Work out the finished part from the listing and answer in its coordinate system (mm). A direction names the side the tool comes from. Coordinates: 2 decimals unless noted, no trailing zeros. Order: outer loops, then holes, each group sorted by start corner. A loop starts at its lowest first (then second) coordinate and runs counter-clockwise, first axis right, second up. Notation, with made-up numbers: M 76.25,-14.5 L 93.25,-14.5 A29 cw 93.25,21.5 Z; hole C 29.25,46.25 d11. An arc over 180 degrees is marked long. Write item = value, one per line. Start each with the question number.
Q1. Determine the mould class of faces 5 (the flat face through (0, 28, 0)), 6 (the flat face through (0, 1000, -290)), 7 (the flat face through (0, 17, 10)) for opening direction Z: released by +Z, released by -Z, zero draft, split by the parting line, or undercut.
Q2. Straight lines are drawn through the part: line 1 along Y through (x, z) = (1.5, 45); line 2 along Z through (x, y) = (-6, 830); line 3 along Z through (x, y) = (-2, 25.5). For each, find the intervals that lie inside material, in ascending order.
Q3. Each of these flat-tipped pins is pushed along its axis until it touches: P1, Ø15, axis at x = 4.5, y = 21, coming from the +Z side; P2, Ø5, axis at x = 0.5, z = 18.5, coming from the +Y side; P3, Ø25, axis at x = 0, y = 38.5, coming from the -Z side; P4, Ø8, axis at x = -15.5, z = 32.5, coming from the -Y side. Where does it stop, or does it pass through?
Q4. Find section A-A on y = 872. Give the vertices of the cut face in (x, z), and give its area (3 significant figures).
Q5. Find section B-B on z = -135.5. Give the vertices of the cut face in (x, y).
Q6. A tool of negligible diameter and unlimited length cuts with its end or side. For faces 1 (the cylindrical face through (-2.17, 523.42, -280.24)), 2 (the cylindrical face through (5.38, 73.43, 39.58)), 3 (the cylindrical face through (-2.17, -9.76, -116.61)), 4 (the cylindrical face through (-0.55, -24.994, 4.93)), from which of +Z, -Z, +X, -X, +Y, -Y can it reach the whole face along a straight path? Write none if from no direction.
```python
from build123d import *

# Parameters (mm, degrees)
SKETCH1_R           = 10
BOSS_EXTRUDE1_DEPTH = 10
SKETCH2_R           = 10
BOSS_EXTRUDE2_DEPTH = 60
SWEEP1_START        = 59.9999999
SWEEP1_OUTLINE_R    = 10
SWEEP1_DEPTH        = 940.0000001
SWEEP1_START_2      = -230.0000001
SWEEP1_2_OUTLINE_R  = 10
SWEEP1_2_DEPTH      = 240.0000001
SWEEP1_3_OUTLINE_R  = 10
SWEEP1_3_ANGLE      = 90


with BuildPart() as part:
    # Sketch1 → Boss-Extrude1 (new body)
    with BuildSketch(Plane.XY):
        with BuildLine():
            ThreePointArc((15, 65), (0, 80), (-15, 65))
            Line((-15, 65), (-23.843930636, 7.514450867))
            Line((-23.843930636, 7.514450867), (-25, 0))
            ThreePointArc((-25, 0), (0, -25), (25, 0))
            Line((25, 0), (23.843930636, 7.514450867))
            Line((23.843930636, 7.514450867), (15, 65))
        make_face()
        Circle(SKETCH1_R, mode=Mode.SUBTRACT)
    extrude(amount=BOSS_EXTRUDE1_DEPTH)

    # Sketch2 → Boss-Extrude2 (add)
    with BuildSketch(Plane.XY.offset(10)):
        with Locations((0, 65)):
            Circle(SKETCH2_R)
    extrude(amount=BOSS_EXTRUDE2_DEPTH)

    # Sweep1 2 outline → Sweep1 2 (add)
    with BuildSketch(Plane.XY.offset(SWEEP1_START_2)):
        Circle(SWEEP1_2_OUTLINE_R)
    extrude(amount=SWEEP1_2_DEPTH)



with BuildPart() as body_2:
    # Sweep1: read off the stored shape, not the designer's step
    # Sweep1 outline → Sweep1 (new body)
    with BuildSketch(Plane(origin=(0, 0, 0), x_dir=(1, 0, 0), z_dir=(0, 1, 0)).offset(SWEEP1_START)):
        with Locations((0, 290)):
            Circle(SWEEP1_OUTLINE_R)
    extrude(amount=SWEEP1_DEPTH)


with BuildPart() as part_1:
    add(part.part)

    add(body_2.part)  # Sweep1 3 merges body 2
    # Sweep1 3 outline → Sweep1 3 (revolve)
    with BuildSketch(Plane(origin=(0, 60, -230), x_dir=(0, -1, 0), z_dir=(0, 0, 1))):
        with Locations((60, 0)):
            Circle(SWEEP1_3_OUTLINE_R)
    revolve(axis=Axis((0, 60, -230), (1, 0, 0)), revolution_arc=SWEEP1_3_ANGLE)


solid = part_1.part
```
Findings below:
q1.face_5 = undercut
q1.face_6 = zero draft
q1.face_7 = released by +Z
q2.line_1 = 55.11 to 74.89
q2.line_2 = -298 to -282
q2.line_3 = -290.68 to -266.47, 0 to 10
q3.P1 = 10
q3.P2 = 75
q3.P3 = -299.42
q3.P4 = through
q4.outline = C 0,-290 d20
q4.area = 314 mm^2
q5.outline = C 0,0 d20
q6.face_1 = +Y
q6.face_2 = +Z
q6.face_3 = none
q6.face_4 = +Z, -Z, -Y
